Input: part model. Units: mm. Frame: model coordinates. A direction names the side the tool comes from. Round coordinates to 2 decimals unless told otherwise and drop trailing zeros. Order: outer loops, then holes, each group sorted by start corner. A loop starts at its lowest first (then second) coordinate and runs counter-clockwise, first axis right, second up. Notation, with made-up numbers: (32.25, 15) -> (60.25, 15) arc R27 cw to (60.25, 41) -> close; hole circle Ø11 at (0.5, -39). An arc over 180 degrees is marked (long way). Use a Markdown table: item, result.
Solid Edge part; units mm, degrees
sketch "Sketch1" plane through (0, 0, 0) normal (0, -1, 0) x (1, 0, 0)
  circle A0 centre (0, 0) radius 3.35
extrude "Protrusion1" add sketch "Sketch1" against normal blind 4
sketch "Sketch2" plane through (0, 4, 0) normal (0, 1, 0) x (-1, 0, 0)
  circle A0 centre (0, 0) radius 2
extrude "ExtrudedProtrusion_2" add sketch "Sketch2" along normal blind 12
fillet "Round_1" radius 0.2 1 edges at (-3.35, 0, 0)
sketch "Sketch3" plane through (0, 0, 0) normal (0, -1, 0) x (1, 0, 0)
  line L0 (0, 1.4434) -> (-1.25, 0.7217)
  line L1 (-1.25, 0.7217) -> (-1.25, -0.7217)
  line L2 (-1.25, -0.7217) -> (0, -1.4434)
  line L3 (0, -1.4434) -> (1.25, -0.7217)
  line L4 (1.25, -0.7217) -> (1.25, 0.7217)
  line L5 (1.25, 0.7217) -> (0, 1.4434)
extrude "ExtrudedCutout_2" cut sketch "Sketch3" against normal blind 2.3
properties material "Steel"
1) Pull-direction query (Z, two-part tool) for faces 1 (the cylindrical face through (0, 10, 2)), 2 (the flat face through (0, 16, 0)), 3 (the flat face through (1.25, 1, 0)), 4 (the flat face through (0.63, 1.13, 1.08)); classes: +Z half, -Z half, draft (parallel to the pull), parting line (faces both ways), or undercut.
Results found:
| item | result |
|---|---|
| face 1 | parting line |
| face 2 | draft |
| face 3 | undercut |
| face 4 | undercut |
2) Cut plane A-A on y = 1.25. Return loops of the section in (x, z).
Results found:
| item | result |
|---|---|
| outline | circle Ø6.7 at (0, 0); hole (-1.25, -0.72) -> (0, -1.44) -> (1.25, -0.72) -> (1.25, 0.72) -> (0, 1.44) -> (-1.25, 0.72) -> close |
3) Line query: L1, parallel to Y at x = 2, z = -1.25; L2, parallel to Z at x = 0, y = 12; L3, parallel to X at y = 0.5, z = -1. Output: solid intervals per line, ascending. Write a range as [from, to].
Results found:
| item | result |
|---|---|
| L1 | y = [0, 4] |
| L2 | z = [-2, 2] |
| L3 | x = [-3.2, -0.77], [0.77, 3.2] |
4) Set-up query: faces 5 (the flat face through (-0.63, 1.13, -1.08)), 6 (the flat face through (-2.2, 4, 0)), 7 (the cylindrical face through (-3.347, 2.073, 0.147)). Return all of +Z, -Z, +X, -X, +Y, -Y with unobstructed straight access to the full face (end or side cutting, diameter ignored); none if empty.
Results found:
| item | result |
|---|---|
| face 5 | -Y |
| face 6 | +Y |
| face 7 | +Y, -Y |
5) Cut plane B-B on y = 10. Return loops of the section in (x, z), and give its area (3 significant figures).
Results found:
| item | result |
|---|---|
| outline | circle Ø4 at (0, 0) |
| area | 12.6 mm² |
6) Pin query (flat end, axial travel): pin 1 Ø1.5 at (y, z) = (2.5, 1) entering from +X; pin 2 Ø4 at (x, y) = (-2.5, 7) entering from -Z; pin 3 Ø1.5 at (x, y) = (-1, 4.5) entering from -Z. Return the tip coordinate at first contact, or that it passes through.
Results found:
| item | result |
|---|---|
| pin 1 | stops at x = 3.34 |
| pin 2 | stops at z = -1.94 |
| pin 3 | stops at z = -3.32 |
